Check sheet for the drawn part. Datum: minimum x, y, z corner. Units: mm. A direction names the side the tool comes from. Round coordinates to 2 decimals unless told otherwise and drop trailing zeros. Order: outer loops, then holes, each group sorted by start corner. A loop starts at its lowest first (then second) coordinate and runs counter-clockwise, first axis right, second up. Notation, with made-up numbers: M -5,-30.75 L 11,-30.75 A15 cw 11,-4.75 Z; hole C 61.5,12.25 d9. An arc over 180 degrees is marked long. Write item = value, one per line. Start each with the question number.
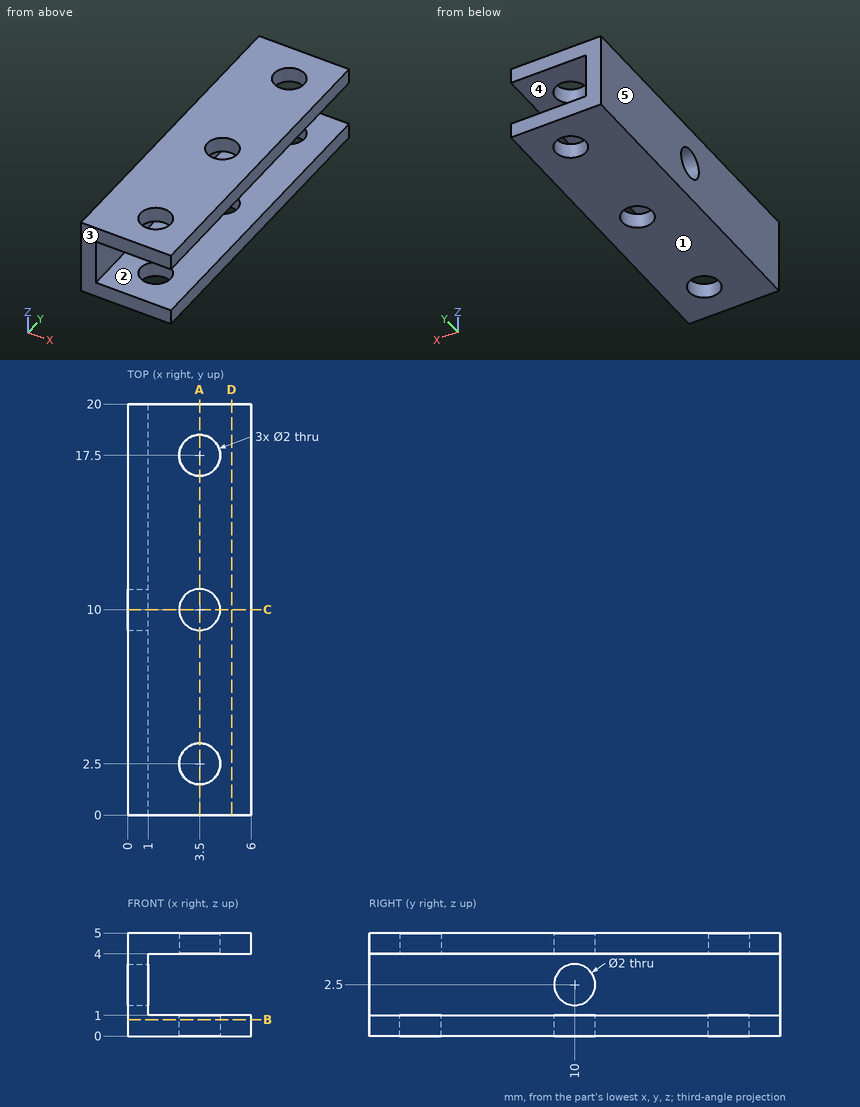
1) Cross-section at D-D, the plane x = 5.05. Enter the section's corners in (y, z).
2) Scan lines: probe 1 along Z at (x, y) = (3.45, 1.25); probe 2 along Y at (x, z) = (3.5, 0.3); probe 3 along Y at (x, z) = (4.1, 0.7). Record each from-to range of solid material in increasing order.
3) Cross-section at B-B, the plane z = 0.8. Enter the section's corners in (x, y), then the cut area to 3 significant figures.
4) Gauge pin test, flat ends, axial feed: P1, Ø2.5, axis at x = 3.5, y = 17.5, coming from the -Z side; P2, Ø0.9, axis at y = 9, z = 2.5, coming from the +X side; P3, Ø1.6, axis at y = 10, z = 2.5, coming from the -X side. Record the tip position at first contact, or that the pin passes through.
5) Cross-section at A-A, the plane x = 3.5. Give the number of separate pieces and of enclosed holes in the cut face, then the cut area to 3 significant figures.
6) Cross-section at C-C, the plane y = 10. Enter the section's corners in (x, z).
7) Access from +Z, -Z, +X, -X, +Y, -Y to the whole of each face (thin tool, end or side, straight path). Record for the marked faces 4 and 5.
8) Release check for a two-part mould opening along Z. For the marked faces 1, 2 and 3 record: pulls with the +Z half, pulls with the -Z half, needs draft (parallel to the pull), parting line crosses it, or undercut.
Geometry results:
q1.outline = M 0,0 L 20,0 L 20,1 L 0,1 Z; M 0,4 L 20,4 L 20,5 L 0,5 Z
q2.probe_1 = 0 to 1, 4 to 5
q2.probe_2 = 0 to 1.5, 3.5 to 9, 11 to 16.5, 18.5 to 20
q2.probe_3 = 0 to 1.7, 3.3 to 9.2, 10.8 to 16.7, 18.3 to 20
q3.outline = M 0,0 L 6,0 L 6,20 L 0,20 Z; hole C 3.5,2.5 d2; hole C 3.5,10 d2; hole C 3.5,17.5 d2
q3.area = 111 mm^2
q4.P1 = 0
q4.P2 = 1
q4.P3 = through
q5.separate_pieces = 8
q5.enclosed_holes = 0
q5.area = 28.0 mm^2
q6.outline = M 0,0 L 2.5,0 L 2.5,1 L 1,1 L 1,1.5 L 0,1.5 Z; M 0,3.5 L 1,3.5 L 1,4 L 2.5,4 L 2.5,5 L 0,5 Z; M 4.5,0 L 6,0 L 6,1 L 4.5,1 Z; M 4.5,4 L 6,4 L 6,5 L 4.5,5 Z
q7.face_4 = +X, +Y, -Y
q7.face_5 = +Z, -Z, -X, +Y, -Y
q8.face_1 = pulls with the -Z half
q8.face_2 = undercut
q8.face_3 = needs draft
